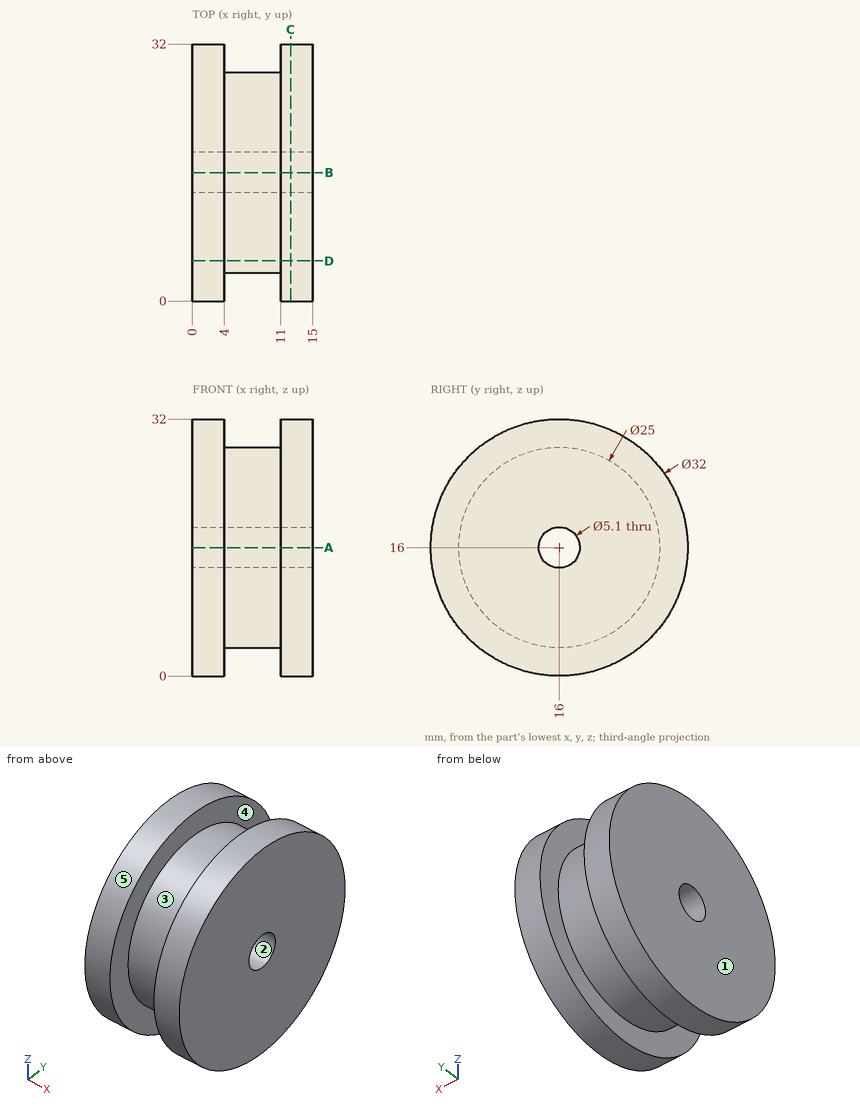
The drawing under review shows one solid part. Ordinate dimensions are in mm from its lowest x, y, z. A direction names the side the tool comes from. Coordinates: 2 decimals unless noted, no trailing zeros. Loops run counter-clockwise (first coordinate to the right, second up) from the corner with the lowest first, then second, coordinate; pieces in that order, holes last.
Item 1: Clearance check with flat-ended pins moving along their axes: pin 1 (6 mm diameter, centred on x = 10, z = 11, fed in from -Y); pin 2 (2 mm diameter, centred on x = 9.5, y = 23, fed in from -Z); pin 3 (5 mm diameter, centred on x = 10, z = 24, fed in from -Y). State where each tip first meets the part, or that it passes through.
Completed:
pin 1: stops at y = 0.15
pin 2: stops at z = 5.03
pin 3: stops at y = 1.05
Item 2: Add section C-C (x = 12.25). Write out the cut boundary in (y, z).
Completed:
outline: circle Ø32 at (16, 16); hole circle Ø5.1 at (16, 16)
Item 3: Wall thickness on L1, parallel to Y at x = 13.75, z = 16; L2, parallel to X at y = 30, z = 15.5; L3, parallel to Y at x = 4.25, z = 16: over which ranges is each line inside the solid? List them lowest first.
Completed:
L1: y = 0 to 13.45, 18.55 to 32
L2: x = 0 to 4, 11 to 15
L3: y = 3.5 to 13.45, 18.55 to 28.5
Item 4: Draft analysis for pull direction X (two halves, no side actions). For the marked faces 1, 2 and 3, state which applies: pulls with the +X half, pulls with the -X half, needs draft (parallel to the pull), parting line crosses it, or undercut.
Completed:
face 1: pulls with the -X half
face 2: needs draft
face 3: undercut
Item 5: Add section A-A (z = 16). Write out the cut boundary in (x, y), and give its area (4 significant figures).
Completed:
outline: (0, 0) - (4, 0) - (4, 3.5) - (11, 3.5) - (11, 0) - (15, 0) - (15, 13.45) - (0, 13.45) - close; (0, 18.55) - (15, 18.55) - (15, 32) - (11, 32) - (11, 28.5) - (4, 28.5) - (4, 32) - (0, 32) - close
area: 354.5 mm2
Item 6: For the marked faces 4 and 5, list the 3-axis set-ups (+Z, -Z, +X, -X, +Y, -Y) from which the entire face can be reached by the end or side of a thin tool; tool diameter is ignored.
Completed:
face 4: none
face 5: +X, -X
Item 7: Add section D-D (y = 5). Write out the cut boundary in (x, z).
Completed:
outline: (0, 4.38) - (4, 4.38) - (4, 10.06) - (11, 10.06) - (11, 4.38) - (15, 4.38) - (15, 27.62) - (11, 27.62) - (11, 21.94) - (4, 21.94) - (4, 27.62) - (0, 27.62) - close
